Could you check a few things on this model? Use its own coordinates, in mm. A direction names the side the tool comes from. Round coordinates to 2 decimals unless told otherwise and drop trailing zeros. Write each loop counter-clockwise with the first axis right and the second up, starting at its lowest first coordinate (ties: lowest second). Pieces come first, ordered by that corner, then holes. Notation, with made-up numbers: (-29, 54) -> (-19, 54) arc R15 ccw to (-19, 77) -> close; hole circle Ø6 at (-21.75, -18). An arc over 180 degrees is marked (long way). Answer as CSV lines item,"result". Start each with the question number.
Q1. Imagine slicing it at C-C on y = 20. Please give me the cut outline in (x, z), and give its area (3 significant figures).
Q2. For faces 4 (the flat face through (0.2, 50, -5.4)), 5 (the flat face through (12.3, 11, 4.3)), 6 (the flat face through (12.3, 5, 4.3)), which set-ups out of +Z, -Z, +X, -X, +Y, -Y let a thin tool reach every point of the face, with its end or its side?
Q3. If we mould it in two halves opening along Z, with no side actions, what happens to faces 1 (the cylindrical face through (-15.569, 8.718, -13.867)), 2 (the flat face through (18, 8, 0)), 3 (the flat face through (0, 8, 18))? For each: pulls with the +Z half, pulls with the -Z half, needs draft (parallel to the pull), parting line crosses it, or undercut.
Q4. Will these pins go through, and if not, where does the flat tip stop? pin 1 Ø5 at (x, z) = (9, 12.5) entering from -Y; pin 2 Ø4 at (x, z) = (12.02, 12.02) entering from -Y; pin 3 Ø3 at (x, y) = (-5, 27) entering from -Z; pin 4 Ø4 at (x, z) = (12.5, 12.5) entering from +Y.
Q5. If I drill on line 1 (Z direction, x = 0, y = 41.5); line 2 (X direction, y = 9, z = -13.5); line 3 (Z direction, x = -4.5, y = 21), over which ranges is the centre line in solid material (lowest first)? Write a range as [from, to].
Q6. Imagine slicing it at A-A on x = 0. Please give me the cut outline in (y, z), and give its area (3 significant figures).
Q7. Imagine slicing it at B-B on z = 0. Please give me the cut outline in (x, y), and give its area (3 significant figures).
Q8. Imagine slicing it at D-D on z = 10.5. Please give me the cut outline in (x, y).
Autodesk Inventor part; units mm, degrees
ref_plane "YZ Plane" through (0, 0, 0) normal (1, 0, 0) x (0, 1, 0)
ref_plane "XZ Plane" through (0, 0, 0) normal (0, 1, 0) x (-1, 0, 0)
ref_plane "XY Plane" through (0, 0, 0) normal (0, 0, 1) x (1, 0, 0)
sketch "Esboço1" plane through (0, 0, 0) normal (0, 0, 1) x (1, 0, 0)
  line L0 (0, 0) -> (0, 50)
  line L1 (-8.5, 0) -> (-8.5, 37)
  line L2 (-8.5, 37) -> (-5, 37)
  line L3 (-5, 37) -> (-5, 50)
  line L4 (-8.5, 0) -> (-12.5, 0)
  line L5 (-12.5, 0) -> (-12.5, 5)
  line L6 (-12.5, 5) -> (-22, 5)
  line L7 (-22, 5) -> (-22, 11)
  line L8 (-22, 11) -> (-12.5, 11)
  line L9 (-12.5, 11) -> (-12.5, 50)
  line L10 (-12.5, 50) -> (-5, 50)
  dimension "d0" = 50
  dimension "d1" = 17
  dimension "d2" = 10
  dimension "d3" = 13
  dimension "d4" = 25
  dimension "d5" = 44
  dimension "d6" = 5
  dimension "d7" = 6
revolve "Revolução1" add sketch "Esboço1" angle 360 about axis through (0, 0, 0) along (0, 1, 0)
sketch "Esboço2" plane through (0, 11, 0) normal (0, 1, 0) x (1, 0, 0)
  circle A0 centre (0, 0) radius 22
  circle A1 centre (0, 0) radius 12.5
  line L0 (-12.6491, 18) -> (12.6491, 18)
  arc A2 (12.6491, 18) -> (-12.6491, 18) centre (0, 0) ccw
  dimension "d9" = 18
extrude "Extrusão1" cut sketch "Esboço2" against normal up to next contours L0 A0 picked at (-0.8962, 19.2784)
pattern_circular "Padrão circular1" count 4 over 360 about axis through (0, -10, 0) along (0, 1, 0) of "Extrusão1"
sketch "Esboço3" plane through (-12.6491, 11, -18) normal (0, 1, 0) x (1, 0, 0)
  circle A0 centre (12.6491, -18) radius 12.5
  line L0 (24.6699, -30.0208) -> (12.6491, -18)
  line L1 (12.6491, -18) -> (30.6491, -18)
  line L2 (30.6491, -5.3509) -> (30.6491, -30.6491)
  dimension "d15" = 45
  dimension "d16" = 17
hole "Furo1" at (12.0208, 11, 12.0208) direction (0, -1, 0) diameter 4.5 end through all counterbore diameter 8 counterbore depth 4.5
pattern_circular "Padrão circular2" count 4 over 360 about axis through (0, -10, 0) along (0, 1, 0) of "Furo1"
Checks:
1,outline,"circle Ø25 at (0, 0); hole circle Ø17 at (0, 0)"
1,area,"264 mm^2"
2,face 4,"+Z, -Z, +X, -X, +Y"
2,face 5,"+Y"
2,face 6,"-Y"
3,face 1,"undercut"
3,face 2,"needs draft"
3,face 3,"pulls with the +Z half"
4,pin 1,"y = 5"
4,pin 2,"through"
4,pin 3,"z = -12"
4,pin 4,"y = 6.5"
5,line 1,"[-12.5, -5], [5, 12.5]"
5,line 2,"[-17.37, -15.74], [-8.3, 8.3], [15.74, 17.37]"
5,line 3,"[-11.66, -7.21], [7.21, 11.66]"
6,outline,"(0, -12.5) -> (5, -12.5) -> (5, -18) -> (11, -18) -> (11, -12.5) -> (50, -12.5) -> (50, -5) -> (37, -5) -> (37, -8.5) -> (0, -8.5) -> close; (0, 8.5) -> (37, 8.5) -> (37, 5) -> (50, 5) -> (50, 12.5) -> (11, 12.5) -> (11, 18) -> (5, 18) -> (5, 12.5) -> (0, 12.5) -> close"
6,area,"557 mm^2"
7,outline,"(-18, 5) -> (-12.5, 5) -> (-12.5, 0) -> (-8.5, 0) -> (-8.5, 37) -> (-5, 37) -> (-5, 50) -> (-12.5, 50) -> (-12.5, 11) -> (-18, 11) -> close; (5, 37) -> (8.5, 37) -> (8.5, 0) -> (12.5, 0) -> (12.5, 5) -> (18, 5) -> (18, 11) -> (12.5, 11) -> (12.5, 50) -> (5, 50) -> close"
7,area,"557 mm^2"
8,outline,"(-18, 5) -> (-13.68, 5) -> (-13.68, 6.5) -> (-15.72, 6.5) -> (-15.72, 11) -> (-18, 11) -> close; (-10.36, 5) -> (-6.78, 5) -> (-6.78, 0) -> (6.78, 0) -> (6.78, 5) -> (10.36, 5) -> (10.36, 6.5) -> (8.32, 6.5) -> (8.32, 11) -> (6.78, 11) -> (6.78, 50) -> (-6.78, 50) -> (-6.78, 11) -> (-8.32, 11) -> (-8.32, 6.5) -> (-10.36, 6.5) -> close; (13.68, 5) -> (18, 5) -> (18, 11) -> (15.72, 11) -> (15.72, 6.5) -> (13.68, 6.5) -> close"
